For this review, take the finished solid that the model builds, in its own axes (mm). Face numbers are marked on the shaded views. Round coordinates to 2 decimals unless told otherwise and drop trailing zeros. Write each loop counter-clockwise with the first axis right and the second up, starting at its lowest first coordinate (ties: lowest second). Pieces come first, ordered by that corner, then holes.
from build123d import *

# Parameters (mm, degrees)
SKETCH1_W           = 100
SKETCH1_H           = 97
BOSS_EXTRUDE1_DEPTH = 3
SKETCH2_W           = 100
SKETCH2_H           = 102
SKETCH2_R           = 37
BOSS_EXTRUDE2_DEPTH = 3


with BuildPart() as part:
    # Sketch1 → Boss-Extrude1 (new body)
    with BuildSketch(Plane(origin=(0, 0, 0), x_dir=(1, 0, 0), z_dir=(0, 1, 0))):
        with Locations((50, 48.5)):
            Rectangle(SKETCH1_W, SKETCH1_H)
        with BuildLine():
            Line((18, 84), (18, 13))
            ThreePointArc((18, 13), (15, 10), (12, 13))
            Line((12, 13), (12, 84))
            ThreePointArc((12, 84), (15, 87), (18, 84))
        make_face(mode=Mode.SUBTRACT)
        with BuildLine():
            Line((82, 13), (82, 84))
            ThreePointArc((82, 84), (85, 87), (88, 84))
            Line((88, 84), (88, 13))
            ThreePointArc((88, 13), (85, 10), (82, 13))
        make_face(mode=Mode.SUBTRACT)
    extrude(amount=BOSS_EXTRUDE1_DEPTH)

    # Sketch2 → Boss-Extrude2 (add)
    with BuildSketch(Plane(origin=(0, 0, -97), x_dir=(-1, 0, 0), z_dir=(0, 0, -1))):
        with Locations((-50, 51)):
            Rectangle(SKETCH2_W, SKETCH2_H)
        with Locations((-50, 59)):
            Circle(SKETCH2_R, mode=Mode.SUBTRACT)
    extrude(amount=-BOSS_EXTRUDE2_DEPTH)


solid = part.part
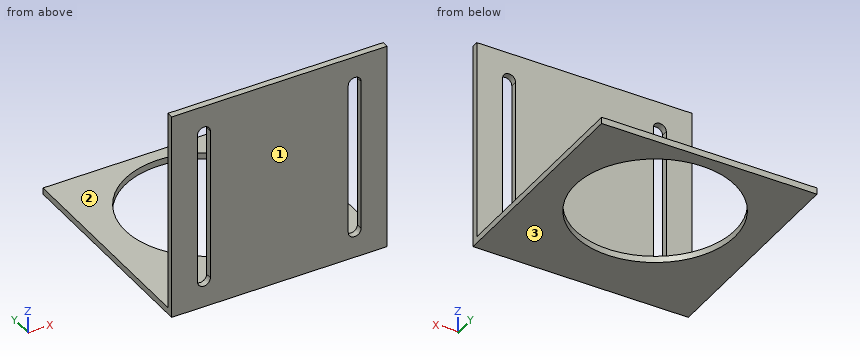
(1) We need section B-B, the plane y = 94. Give the boundary of the cut face in (x, z), and give its area (3 significant figures).
Geometry check:
outline: (0, -97) - (38, -97) - (38, -94) - (0, -94) - close; (62, -97) - (100, -97) - (100, -94) - (62, -94) - close
area: 228 mm2
(2) Mouldability with a two-part tool opening along Z and no side actions: class the marked faces 1, 2 and 3 as pulls with the +Z half, pulls with the -Z half, needs draft (parallel to the pull), parting line crosses it, or undercut.
Geometry check:
face 1: needs draft
face 2: pulls with the +Z half
face 3: pulls with the -Z half
(3) For pin 1 Ø1.5 at (y, z) = (1, -49) entering from -X; pin 2 Ø10 at (x, z) = (19.5, -41.5) entering from +Y, all flat-tipped, find the tip position at first contact; note any pin that passes through.
Geometry check:
pin 1: stops at x = 0
pin 2: stops at y = 3
(4) We need section C-C, the plane x = 85. Give the boundary of the cut face in (y, z).
Geometry check:
outline: (0, -97) - (47, -97) - (47, -94) - (3, -94) - (3, -87) - (0, -87) - close; (0, -10) - (3, -10) - (3, 0) - (0, 0) - close; (71, -97) - (102, -97) - (102, -94) - (71, -94) - close
(5) We need section A-A, the plane z = -27. Give the boundary of the cut face in (x, y).
Geometry check:
outline: (0, 0) - (12, 0) - (12, 3) - (0, 3) - close; (18, 0) - (82, 0) - (82, 3) - (18, 3) - close; (88, 0) - (100, 0) - (100, 3) - (88, 3) - close
(6) We need section D-D, the plane x = 50. Give the boundary of the cut face in (y, z).
Geometry check:
outline: (0, -97) - (22, -97) - (22, -94) - (3, -94) - (3, 0) - (0, 0) - close; (96, -97) - (102, -97) - (102, -94) - (96, -94) - close
(7) For line 1 along Y through (x, z) = (50, -95); line 2 along Z through (x, y) = (7, 88); line 3 along Y through (x, z) = (38, -15), list the stretches that pass through material, from the lowest coordinate up.
Geometry check:
line 1: y = 0 to 22, 96 to 102
line 2: z = -97 to -94
line 3: y = 0 to 3
